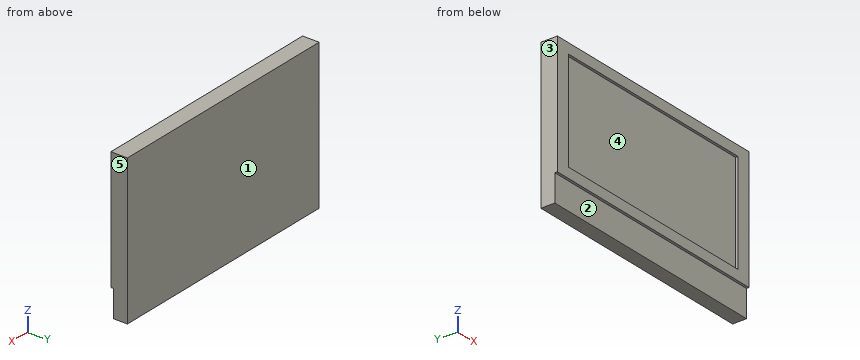
from build123d import *

# Parameters (mm, degrees)
F1_W     = 141.67
F1_H     = 70.844
F1_H_2   = 15.791
F2_DEPTH = 8.14
F3_W     = 125.39
F3_H     = 58.984
F4_DEPTH = 1.5
F5_SCALE = 0.566


with BuildPart() as f2:
    # F1 (on Front) → F2 (new body)
    with BuildSketch(Plane.XZ):
        with Locations((70.835, 51.213)):
            Rectangle(F1_W, F1_H)
        with Locations((70.835, 7.8955)):
            Rectangle(F1_W, F1_H_2)
    extrude(amount=F2_DEPTH)

    # F3 (on offset) → F4 (join)
    with BuildSketch(Plane.XZ.offset(8.14)):
        Polygon((0, 86.635), (0, 15.791), (141.67, 15.791), (141.67, 21.721), (141.67, 80.705), (141.67, 86.635), (133.53, 86.635), (8.14, 86.635), align=None)
        with Locations((70.835, 51.213)):
            Rectangle(F3_W, F3_H, mode=Mode.SUBTRACT)
    extrude(amount=F4_DEPTH)


with BuildPart() as f2_1:
    # F5: moved
    add(f2.part.scale(F5_SCALE))


solid = f2_1.part
Read the model definition and answer for the solid it produces. Units are mm, in the model's axes. Face numbers are marked on the shaded views. A direction names the side the tool comes from. Round coordinates to 2 decimals unless told otherwise and drop trailing zeros. Loops run counter-clockwise (first coordinate to the right, second up) from the corner with the lowest first, then second, coordinate; pieces in that order, holes last.
Q1. Section A-A on z = 34.5 is taken. Write down the section's boundary in (x, y).
Q2. Section C-C on z = 8 is taken. Write down the section's boundary in (x, y).
Q3. Section B-B on x = 73.5 is taken. Write down the section's boundary in (y, z).
Q4. Consider probe 1 along Z at (x, y) = (43, -4.8); probe 2 along X at (y, z) = (-4.7, 28); probe 3 along Y at (x, z) = (47, 22.5). Determine where each line is inside the solid, lowest interval first.
Q5. Which of the six approach directions +Z, -Z, +X, -X, +Y, -Y give full straight-line access (tool end or side, diameter ignored) to the marked faces 1 and 2?
Q6. Determine the mould class of the marked faces 3, 4 and 5 for opening direction X: released by +X, released by -X, zero draft, split by the parting line, or undercut.
Output:
1. outline: (0, -5.46) - (4.61, -5.46) - (4.61, -4.61) - (75.58, -4.61) - (75.58, -5.46) - (80.19, -5.46) - (80.19, 0) - (0, 0) - close
2. outline: (0, -4.61) - (80.19, -4.61) - (80.19, 0) - (0, 0) - close
3. outline: (-5.46, 8.94) - (-4.61, 8.94) - (-4.61, 0) - (0, 0) - (0, 49.04) - (-5.46, 49.04) - (-5.46, 45.68) - (-4.61, 45.68) - (-4.61, 12.29) - (-5.46, 12.29) - close
4. probe 1: z = 8.94 to 12.29, 45.68 to 49.04
4. probe 2: x = 0 to 4.61, 75.58 to 80.19
4. probe 3: y = -4.61 to 0
5. face 1: +Z, -Z, +X, -X, +Y
5. face 2: -Z, +X, -X, -Y
6. face 3: released by -X
6. face 4: undercut
6. face 5: released by +X
